from build123d import *

# Parameters (mm, degrees)
CYLINDER001_R     = 22
CYLINDER001_DEPTH = 20
BOX_W             = 10
BOX_H             = 25
BOX_DEPTH         = 10
ARRAY_COUNT       = 8
CYLINDER_R        = 30
CYLINDER_DEPTH    = 100


with BuildPart() as cilindre001:
    # Cylinder001 → Cylinder001 (new body)
    with BuildSketch(Plane(origin=(1, -17, 80), x_dir=(1, 0, 0), z_dir=(0, 0, 1))):
        Circle(CYLINDER001_R)
    extrude(amount=CYLINDER001_DEPTH)


with BuildPart() as array:
    # Box → Box (new body)
    with BuildSketch(Plane.XY):
        with Locations((5, 12.5)):
            Rectangle(BOX_W, BOX_H)
    extrude(amount=BOX_DEPTH)

    # Array: Array ×8 about axis
    array_axis = Axis((0, -18, 0), (0, 0, 1))


with BuildPart() as array_1:
    add(array.part)
    for i in range(1, ARRAY_COUNT):
        add(array.part.rotate(array_axis, i * 360 / ARRAY_COUNT))


with BuildPart() as array_2:
    # Array placement: moved
    add(array_1.part.moved(Location((0, 0, 90))))


with BuildPart() as cut001:
    # Cylinder → Cylinder (new body)
    with BuildSketch(Plane(origin=(0, -17, 0), x_dir=(1, 0, 0), z_dir=(0, 0, 1))):
        Circle(CYLINDER_R)
    extrude(amount=CYLINDER_DEPTH)

    # Cut: cut Array
    add(array_2.part, mode=Mode.SUBTRACT)

    # Cut001: cut Cilindre001
    add(cilindre001.part, mode=Mode.SUBTRACT)


solid = cut001.part
Verification items for the finished model (mm, model axes). A direction names the side the tool comes from. Coordinates: 2 decimals unless noted, no trailing zeros. Order: outer loops, then holes, each group sorted by start corner. A loop starts at its lowest first (then second) coordinate and runs counter-clockwise, first axis right, second up.
1. Set-up check for faces 4 (the face through (18, -36, 95)), 5 (the face through (10, 7, 95)), 6 (the face through (24, -28, 95)), 7 (the face through (-15, 4, 90)): record each of +Z, -Z, +X, -X, +Y, -Y from which the full face is reachable in a straight line by a thin tool's end or side.
Results found:
face 4: +Z, -Y
face 5: +Z, +Y
face 6: +Z, +X
face 7: +Z
2. Sectioned sample at B-B, the plane z = 60. Record the cut outline in (x, y), and give its area (3 significant figures).
Results found:
outline: circle Ø60 at (0, -17)
area: 2,830 mm2
3. Sectioned sample at D-D, the plane y = 0. Record the cut outline in (x, z), and give its area (3 significant figures).
Results found:
outline: (-24.72, 0) - (24.72, 0) - (24.72, 90) - (18, 90) - (18, 100) - (14.96, 100) - (14.96, 80) - (-12.96, 80) - (-12.96, 90) - (-18, 90) - (-18, 100) - (-24.72, 100) - close
area: 4,270 mm2
4. Go/stop test with flat-tipped pins: pin 1 Ø12 at (x, z) = (-11, 25) entering from -Y; pin 2 Ø1.5 at (x, z) = (-1, 30.5) entering from -Y; pin 3 Ø4 at (y, z) = (7, 94) entering from -X. Record where each tip stops, or that it passes through.
Results found:
pin 1: stops at y = -46.58
pin 2: stops at y = -47
pin 3: stops at x = -12.86
5. Scan lines: line 1 (Y direction, x = 1, z = 86); line 2 (X direction, y = -17, z = 89.75); line 3 (Z direction, x = -2, y = 1). Record each from-to range of solid material in increasing order.
Results found:
line 1: y = -46.98 to -39, 5 to 12.98
line 2: x = -30 to -21, 23 to 30
line 3: z = 0 to 80
6. Sectioned sample at A-A, the plane y = -22.5. Record the cut outline in (x, z), and give its area (3 significant figures).
Results found:
outline: (-29.49, 0) - (29.49, 0) - (29.49, 90) - (22.3, 90) - (22.3, 80) - (-20.3, 80) - (-20.3, 100) - (-29.49, 100) - close
area: 4,970 mm2
7. Release check for a two-part mould opening along X. For faces 1 (the face through (-19, 1, 95)), 2 (the face through (-18, -36, 95)), 3 (the face through (-24, -8, 95)) record: +X half, -X half, draft (parallel to the pull), parting line (faces both ways), or undercut.
Results found:
face 1: undercut
face 2: -X half
face 3: draft
8. Sectioned sample at C-C, the plane y = -13.5. Record the cut outline in (x, z), and give its area (3 significant figures).
Results found:
outline: (-29.8, 0) - (29.8, 0) - (29.8, 100) - (22.72, 100) - (22.72, 80) - (-20.72, 80) - (-20.72, 90) - (-29.8, 90) - close
area: 5,000 mm2
